```python
from build123d import *

# Parameters (mm, degrees)
SKETCH1_R            = 10
BOSS_EXTRUDE1_DEPTH  = 20
SKETCH2_R            = 12.5
BOSS_EXTRUDE2_DEPTH  = 3
FILLET1_R            = 1
FILLET1_OF_MIRROR1_R = 1


with BuildPart() as part:
    # Sketch1 → Boss-Extrude1 (new body)
    with BuildSketch(Plane.XY):
        Circle(SKETCH1_R)
    extrude(amount=BOSS_EXTRUDE1_DEPTH)

    # Sketch2 → Boss-Extrude2 (add)
    with BuildSketch(Plane(origin=(0, 0, 0), x_dir=(-1, 0, 0), z_dir=(0, 0, -1))):
        Circle(SKETCH2_R)
    boss_extrude2 = extrude(amount=BOSS_EXTRUDE2_DEPTH)

    # Fillet1
    fillet1_edges = [part.edges().sort_by_distance(p)[0] for p in [
        (12.5, 0, -3),
    ]]
    fillet(fillet1_edges, radius=FILLET1_R)

    # Mirror1: Boss-Extrude2 across plane
    add(boss_extrude2.mirror(Plane.XY.offset(10)))

    # Fillet1 of Mirror1
    fillet1_of_mirror1_edges = [part.edges().sort_by_distance(p)[0] for p in [
        (12.5, 0, 23),
    ]]
    fillet(fillet1_of_mirror1_edges, radius=FILLET1_OF_MIRROR1_R)


solid = part.part
```
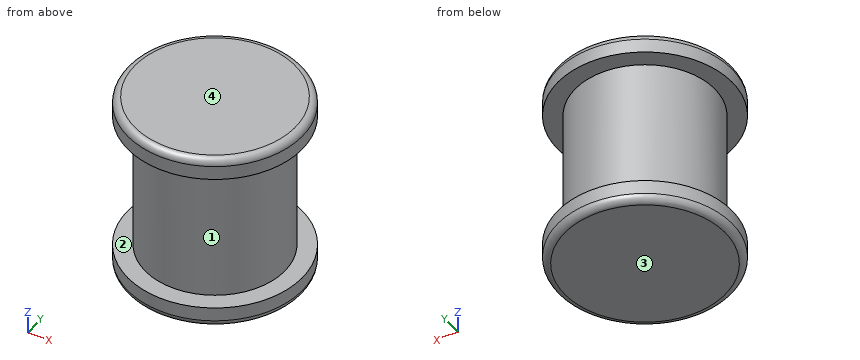
Can you work these out from the model? Positions are in its coordinate system, mm. Face numbers are marked on the shaded views. Coordinates: 2 decimals unless noted, no trailing zeros. Loops run counter-clockwise (first coordinate to the right, second up) from the corner with the lowest first, then second, coordinate; pieces in that order, holes last.
Item 1: I'm going to push flat-ended pins straight in: pin 1 (5 mm diameter, centred on y = 0, z = 11.5, fed in from -X); pin 2 (3 mm diameter, centred on y = -5, z = 7, fed in from -X); pin 3 (1.5 mm diameter, centred on y = -4.5, z = 3, fed in from -X). Where does each tip first touch, or does it pass through?
Answers below:
pin 1: stops at x = -10
pin 2: stops at x = -9.37
pin 3: stops at x = -9.27
Item 2: Suppose I cut it at C-C (z = 10.25). Please give me the cut outline in (x, y).
Answers below:
outline: circle Ø20 at (0, 0)
Item 3: Please list where these lines run through material, in increasing order: L1, parallel to Z at x = 3, y = -11; L2, parallel to X at y = -8.25, z = 4.25; L3, parallel to X at y = 7.75, z = -1.
Answers below:
L1: z = -3 to 0, 20 to 23
L2: x = -5.65 to 5.65
L3: x = -9.81 to 9.81
Item 4: Suppose I cut it at A-A (x = 0). Please give me the cut outline in (y, z), then the cut area to 3 significant figures.
Answers below:
outline: (-12.5, -2) arc R1 ccw to (-11.5, -3) - (11.5, -3) arc R1 ccw to (12.5, -2) - (12.5, 0) - (10, 0) - (10, 20) - (12.5, 20) - (12.5, 22) arc R1 ccw to (11.5, 23) - (-11.5, 23) arc R1 ccw to (-12.5, 22) - (-12.5, 20) - (-10, 20) - (-10, 0) - (-12.5, 0) - close
area: 549 mm2
Item 5: If we mould it in two halves opening along Z, with no side actions, what happens to the marked faces 1, 2, 3 and 4? For each: released by +Z, released by -Z, zero draft, split by the parting line, or undercut.
Answers below:
face 1: undercut
face 2: undercut
face 3: released by -Z
face 4: released by +Z
